```python
from build123d import *

# Parameters (mm, degrees)
F0_W     = 27.7
F0_H     = 25
F1_DEPTH = 10
F2_DEPTH = 10
F3_R     = 5


# Not quite as in the source:
# - a feature names something its author has since deleted; it is built from what else it names


with BuildPart() as f1:
    # F0 (on Top) → F1 (new body)
    with BuildSketch(Plane.XY):
        with BuildLine():
            Line((-18, 25), (-18, 50))
            ThreePointArc((-18, 50), (-43, 25), (-18, 0))
            Line((-18, 0), (-18, 25))
        make_face()
        with BuildLine():
            ThreePointArc((9.7, 25), (22.2, 37.5), (9.7, 50))
            Line((9.7, 50), (9.7, 25))
        make_face()
        with Locations((-4.15, 37.5)):
            Rectangle(F0_W, F0_H)
    extrude(amount=F1_DEPTH)

    # F2 (add): a face of the model
    f2_faces = [f1.faces().sort_by_distance(p)[0] for p in [
        (-14.2102397427, 31.107363361, 10),
    ]]
    extrude(f2_faces, amount=F2_DEPTH)

    # F3
    f3_edges = [f1.edges().sort_by_distance(p)[0] for p in [
        (-4.15, 25, 20),
        (9.7, 25, 10),
        (-4.15, 25, 0),
        (-18, 25, 10),
        (-4.15, 50, 20),
        (22.2, 37.5, 20),
        (-43, 25, 20),
        (-18, 12.5, 20),
        (-18, 50, 10),
        (-18, 0, 10),
        (-43, 25, 0),
        (-18, 12.5, 0),
        (22.2, 37.5, 0),
        (-4.15, 50, 0),
    ]]
    fillet(f3_edges, radius=F3_R)


solid = f1.part
```
Could you check a few things on this model? Use its own coordinates, in mm. A direction names the side the tool comes from. Round coordinates to 2 decimals unless told otherwise and drop trailing zeros. Write each loop counter-clockwise with the first axis right and the second up, starting at its lowest first coordinate (ties: lowest second). Pieces come first, ordered by that corner, then holes. Notation, with made-up numbers: M 28,81 L 37,81 A30 cw 37,114 Z; hole C 84,67.25 d3. An arc over 180 degrees is marked long. Answer in a Markdown table with one row per item. Add a question column.
Q1. If I drill on line 1 (Y direction, x = -6.5, z = 10); line 2 (X direction, y = 45, z = 14); line 3 (X direction, y = 29, z = 16.75), over which ranges is the centre line in solid material (lowest first)? Write a range as from..to.
Q2. Imagine slicing it at A-A (z = 9). Please give me the cut outline in (x, y), then the cut area to 3 significant figures.
Q3. Imagine slicing it at B-B (z = 2.25). Please give me the cut outline in (x, y).
Q4. Will these pins go through, and if not, where does the flat tip stop? pin 1 Ø6 at (y, z) = (18, 9) entering from +X; pin 2 Ø8 at (y, z) = (20, 3) entering from -X; pin 3 Ø11 at (x, z) = (-3, 8) entering from -Y.
Q5. On a 3-axis mill with a long thin cutter (end or side, diameter ignored), from which of +Z, -Z, +X, -X, +Y, -Y can I reach the whole of each face in a straight line? I mean faces 1 (the cylindrical face through (-19, 13, 18)), 2 (the flat face through (-2, 25, 10)), 3 (the cylindrical face through (-20, 13, 1)). Say none if no direction works.
Values:
| question | item | result |
|---|---|---|
| 1 | line 1 | 25..50 |
| 1 | line 2 | -33..19.7 |
| 1 | line 3 | -42.36..18.43 |
| 2 | outline | M -24.25,0.79 A5 ccw -18,5.64 L -18,20 A5 cw -13,25 L 9.7,25 A12.5 ccw 9.7,50 L -18,50 A25 ccw Z |
| 2 | area | 1,920 mm^2 |
| 3 | outline | M -24.04,1.59 A4.18 ccw -18.82,5.64 L -18.82,20 A5.82 cw -13,25.82 L 9.7,25.82 A11.68 ccw 9.7,49.18 L -18,49.18 A24.18 ccw Z |
| 4 | pin 1 | x = -17.9 |
| 4 | pin 2 | x = -42.96 |
| 4 | pin 3 | y = 25 |
| 5 | face 1 | +Z, +X, -Y |
| 5 | face 2 | +Z, -Z, +X, -Y |
| 5 | face 3 | -Z, +X, -Y |
